Geometry: final body of the model. Coordinates: model frame, mm. A direction names the side the tool comes from. Give positions to 0.01 mm unless a question says otherwise; leave off trailing zeros. Order: outer loops, then holes, each group sorted by start corner. A loop starts at its lowest first (then second) coordinate and runs counter-clockwise, first axis right, second up. Notation, with made-up numbers: (45.25, 15.5) -> (104.25, 15.5) arc R32 cw to (104.25, 43.5) -> close; hole circle Ø6 at (37.25, 23). An arc over 180 degrees is marked (long way). One line per question, with ' | ' between items. Start each with the question number.
(1) Section B-B (z = 0). Return loops of the section in (x, y).
(2) Section A-A (y = 0). Return loops of the section in (x, z), then the cut area to 3 significant figures.
(3) Set-up query: faces 1 (the face through (-20.4, 0.4, 24)), 2 (the face through (-23.994, 0.528, 4.488)). Return all of +Z, -Z, +X, -X, +Y, -Y with unobstructed straight access to the full face (end or side cutting, diameter ignored); none if empty.
(4) First-contact query: pin 1 Ø4 at (y, z) = (0, 0) entering from -X; pin 2 Ø8 at (x, z) = (-9, -3) entering from +Y; pin 3 Ø4 at (x, z) = (-13, 12.5) entering from -Y; pin 4 Ø5 at (x, z) = (-16, -13.5) entering from +Y. Flat tips, straight axial feed; report the tip coordinate or a pass-through.
(5) Section C-C (z = 17). Return loops of the section in (x, y), then the cut area to 3 significant figures.
(6) Ray query, L1, parallel to Z at x = -21, y = 0; L2, parallel to Z at x = -20.5, y = 19; L3, parallel to Y at x = -28.5, z = 0. Return the intervals inside material, ascending.
```python
from build123d import *

# Parameters (mm, degrees)
SKETCH_1_R          = 24
SKETCH_1_R_2        = 20
EXTRUDE_1_DEPTH     = 24
SKETCH_2_R          = 29
SKETCH_2_R_2        = 24
EXTRUDE_2_DEPTH     = 5
SKETCH_5_W          = 29
SKETCH_5_H          = 58
CUT_EXTRUDE_1_DEPTH = 49
CHAMFER_2_SIZE      = 1
EXTRUDE_START       = -30
SKETCH_6_R          = 4
SKETCH_6_R_2        = 1.5
EXTRUDE_3_DEPTH     = 6.335681
SKETCH_6_2_R        = 1.5
CUT_EXTRUDE_2_DEPTH = 31.0000001


with BuildPart() as part:
    # Sketch 1 → Extrude 1 (new body)
    with BuildSketch(Plane.XY):
        Circle(SKETCH_1_R)
        Circle(SKETCH_1_R_2, mode=Mode.SUBTRACT)
    extrude(amount=EXTRUDE_1_DEPTH)

    # Sketch 2 → Extrude 2 (add)
    with BuildSketch(Plane.XY.offset(24)):
        Circle(SKETCH_2_R)
        Circle(SKETCH_2_R_2, mode=Mode.SUBTRACT)
    extrude(amount=-EXTRUDE_2_DEPTH)

    # Mirror 1: part across plane


with BuildPart() as part_1:
    add(part.part)
    add(part.part.mirror(Plane.XY))

    # Sketch 5 → Cut-Extrude 1 (cut, through all)
    with BuildSketch(Plane.XY.offset(24)):
        with Locations((14.5, 0)):
            Rectangle(SKETCH_5_W, SKETCH_5_H)
    extrude(amount=-CUT_EXTRUDE_1_DEPTH, mode=Mode.SUBTRACT)

    # Chamfer 2
    chamfer_2_edges = [part_1.edges().sort_by_distance(p)[0] for p in [
        (-29, 0, -24),
        (-29, 0, 24),
    ]]
    chamfer(chamfer_2_edges, length=CHAMFER_2_SIZE)

    # Sketch 6 → Extrude 3 (add)
    with BuildSketch(Plane(origin=(0, 0, 0), x_dir=(0, 0, -1), z_dir=(1, 0, 0)).offset(EXTRUDE_START)):
        Circle(SKETCH_6_R)
        Circle(SKETCH_6_R_2, mode=Mode.SUBTRACT)
    extrude(amount=EXTRUDE_3_DEPTH)

    # Sketch 6_2 → Cut-Extrude 2 (cut, through all)
    with BuildSketch(Plane(origin=(0, 0, 0), x_dir=(0, 0, -1), z_dir=(1, 0, 0))):
        Circle(SKETCH_6_2_R)
    extrude(amount=-CUT_EXTRUDE_2_DEPTH, mode=Mode.SUBTRACT)


solid = part_1.part
```
Response:
1) outline: (-30, -4) -> (-23.66, -4) arc R24 ccw to (0, -24) -> (0, -20) arc R20 cw to (-19.94, -1.5) -> (-30, -1.5) -> close; (-30, 1.5) -> (-19.94, 1.5) arc R20 cw to (0, 20) -> (0, 24) arc R24 ccw to (-23.66, 4) -> (-30, 4) -> close
2) outline: (-30, -4) -> (-24, -4) -> (-24, -19) -> (-29, -19) -> (-29, -23) -> (-28, -24) -> (-20, -24) -> (-20, -1.5) -> (-30, -1.5) -> close; (-30, 1.5) -> (-20, 1.5) -> (-20, 24) -> (-28, 24) -> (-29, 23) -> (-29, 19) -> (-24, 19) -> (-24, 4) -> (-30, 4) -> close | area: 259 mm^2
3) face 1: +Z, +X, -X, +Y, -Y | face 2: -X
4) pin 1: stops at x = -30 | pin 2: stops at y = 23.47 | pin 3: stops at y = -21.33 | pin 4: stops at y = 19.84
5) outline: (0, -24) -> (0, -20) arc R20 cw to (0, 20) -> (0, 24) arc R24 ccw to start | area: 276 mm^2
6) L1: z = -24 to -1.5, 1.5 to 24 | L2: z = -24 to -19, 19 to 24 | L3: y = -4 to -1.5, 1.5 to 4
